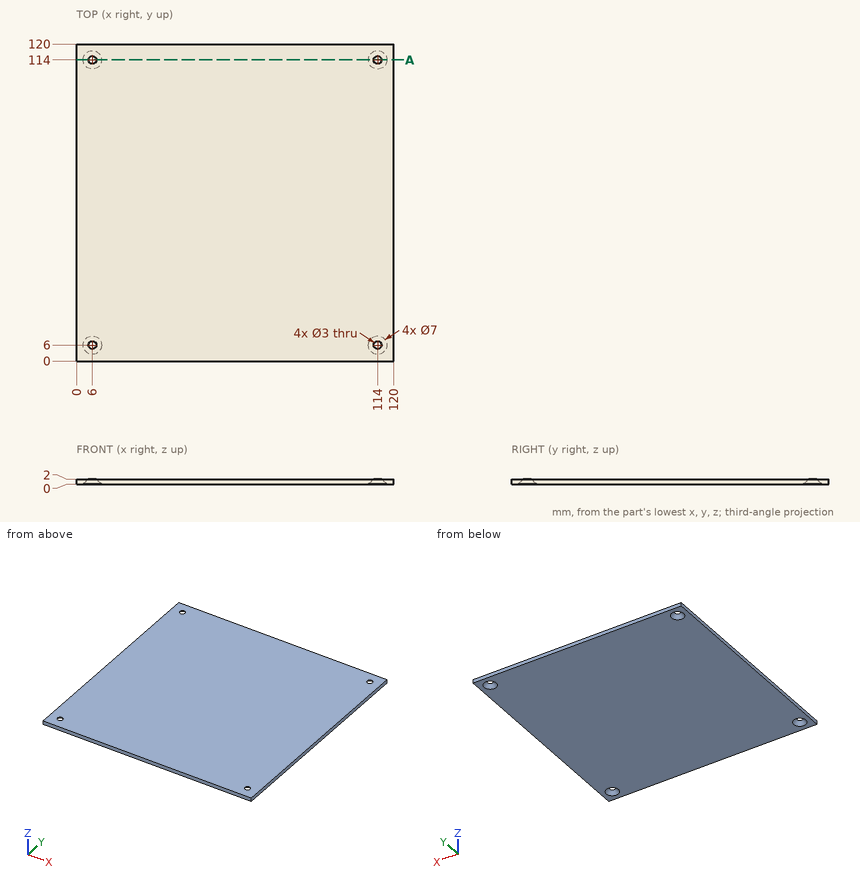
Drawing for the job (mm, zero at the part's lowest x, y, z). Give positions to 0.01 mm unless a question says otherwise; leave off trailing zeros. Return JSON: item names as keys, results as strings. Group by question number.
(1) Flat gauge pin, fed straight in: pin 1 Ø4 at (x, y) = (114, 114) entering from -Z. Where does the tip first touch, or does it go through?
(2) Band-saw the part on A-A (y = 114). State how many separate pieces and enclosed holes the cut face has, and give its area (3 significant figures).
(3) Drill centre line: L1, parallel to Y at x = 8, z = 1.15 (1 decimal). Where is it in solid material? Low to high. Write a range as [from, to].
Entries:
{
 "1": {"pin 1": "stops at z = 1.5"},
 "2": {"separate pieces": "3", "enclosed holes": "0", "area": "220 mm^2"},
 "3": {"L1": "y = [0, 4.8], [7.2, 112.8], [115.2, 120]"}
}
